Check sheet for the modelled part. Datum: model origin and axes. Units: mm. A direction names the side the tool comes from. Round coordinates to 2 decimals unless told otherwise and drop trailing zeros. Write each loop counter-clockwise with the first axis right and the second up, starting at its lowest first coordinate (ties: lowest second). Pieces come first, ordered by that corner, then holes. Notation, with made-up numbers: (0.5, 3) -> (55.5, 3) arc R6 ccw to (55.5, 9) -> close; hole circle Ø5 at (30.25, 17.5). An arc over 180 degrees is marked (long way). Put each result on its own line as item: value. Start each with the question number.
from build123d import *

# Parameters (mm, degrees)
IZIM1_R                     = 45
Y_KSEKLIK_EKSTR_ZYON1_DEPTH = 35
IZIM2_W                     = 34
IZIM2_H                     = 34
KES_EKSTR_ZYON1_DEPTH       = 4
IZIM5_R                     = 12
KES_EKSTR_ZYON2_DEPTH       = 107.536378763
KES_EKSTR_ZYON3_DEPTH       = 19
IZIM8_R                     = 45
IZIM8_R_2                   = 43
KES_EKSTR_ZYON4_DEPTH       = 1.5
KES_EKSTR_ZYON5_REACH       = 108.536
IZIM9_R                     = 1.5
DAIRESEL_KAPLAMA1_COUNT     = 6


with BuildPart() as part:
    # Çizim1 → Yükseklik-Ekstrüzyon1 (new, symmetric)
    with BuildSketch(Plane(origin=(0, 0, 0), x_dir=(1, 0, 0), z_dir=(0, 1, 0))):
        with Locations(Location((0, 0, 0), (0, 0, 270))):
            Circle(IZIM1_R)
    extrude(amount=Y_KSEKLIK_EKSTR_ZYON1_DEPTH, both=True)

    # Çizim2 → Kes-Ekstrüzyon1 (cut)
    with BuildSketch(Plane.XY.offset(45)):
        with Locations((0, -10)):
            Rectangle(IZIM2_W, IZIM2_H)
    kes_ekstr_zyon1 = extrude(amount=-KES_EKSTR_ZYON1_DEPTH, mode=Mode.SUBTRACT)

    # Aynalama1: Kes-Ekstrüzyon1 across plane
    add(kes_ekstr_zyon1.mirror(Plane.XY), mode=Mode.SUBTRACT)

    # Çizim5 → Kes-Ekstrüzyon2 (cut, through all)
    with BuildSketch(Plane.XY.offset(45)):
        with Locations((0, -10)):
            Circle(IZIM5_R)
    extrude(amount=-KES_EKSTR_ZYON2_DEPTH, mode=Mode.SUBTRACT)

    # Çizim7 → Kes-Ekstrüzyon3 (cut, symmetric)
    with BuildSketch(Plane(origin=(0, 0, 0), x_dir=(0, 0, -1), z_dir=(1, 0, 0))):
        with BuildLine():
            Line((38, -35), (38, -27))
            Line((38, -27), (12, -27))
            Line((12, -27), (12, 11))
            Line((12, 11), (38, 11))
            Line((38, 11), (38, 26))
            ThreePointArc((38, 26), (37.414213562, 27.414213562), (36, 28))
            Line((36, 28), (-36, 28))
            ThreePointArc((-36, 28), (-37.414213562, 27.414213562), (-38, 26))
            Line((-38, 26), (-38, 11))
            Line((-38, 11), (-11.999999881, 11))
            Line((-11.999999881, 11), (-11.999999881, -27))
            Line((-11.999999881, -27), (-38, -27))
            Line((-38, -27), (-38, -35))
            Line((-38, -35), (38, -35))
        make_face()
    extrude(amount=KES_EKSTR_ZYON3_DEPTH, both=True, mode=Mode.SUBTRACT)

    # Çizim8 → Kes-Ekstrüzyon4 (cut, symmetric)
    with BuildSketch(Plane(origin=(0, 23.5, 0), x_dir=(1, 0, 0), z_dir=(0, 1, 0))):
        with Locations(Location((0, 0, 0), (0, 0, 270))):
            Circle(IZIM8_R)
        with Locations(Location((0, 0, 0), (0, 0, 270))):
            Circle(IZIM8_R_2, mode=Mode.SUBTRACT)
    extrude(amount=KES_EKSTR_ZYON4_DEPTH, both=True, mode=Mode.SUBTRACT)

    # Çizim9 → Kes-Ekstrüzyon5 (cut, up to next)
    with BuildSketch(Plane.XY.offset(45), mode=Mode.PRIVATE) as kes_ekstr_zyon5_sk1:
        with Locations(Location((0, 23.5, 0), (0, 0, 90))):
            Circle(IZIM9_R)
    kes_ekstr_zyon5_tool1 = extrude(kes_ekstr_zyon5_sk1.sketch, amount=-KES_EKSTR_ZYON5_REACH, mode=Mode.PRIVATE) & part.part
    kes_ekstr_zyon5 = kes_ekstr_zyon5_tool1.solids().sort_by_distance((0, 23.5, 45))[0]
    add(kes_ekstr_zyon5, mode=Mode.SUBTRACT)

    # Dairesel Kaplama1: Kes-Ekstrüzyon5; each copy of Kes-Ekstrüzyon5 runs up to whatever stops it at its own place
    dairesel_kaplama1_before = part.part  # the part as the pattern finds it: every copy runs up to it
    dairesel_kaplama1_kes_ekstr_zyon5_long = extrude(kes_ekstr_zyon5_sk1.sketch, amount=-KES_EKSTR_ZYON5_REACH, mode=Mode.PRIVATE)
    dairesel_kaplama1_kes_ekstr_zyon5_tool = dairesel_kaplama1_kes_ekstr_zyon5_long.rotate(Axis((0, 25, 0), (0, 1, 0)), 1 * 360 / DAIRESEL_KAPLAMA1_COUNT) & dairesel_kaplama1_before
    add(dairesel_kaplama1_kes_ekstr_zyon5_tool.solids().sort_by_distance((38.971143, 23.5, 22.5))[0], mode=Mode.SUBTRACT)
    dairesel_kaplama1_kes_ekstr_zyon5_tool = dairesel_kaplama1_kes_ekstr_zyon5_long.rotate(Axis((0, 25, 0), (0, 1, 0)), 2 * 360 / DAIRESEL_KAPLAMA1_COUNT) & dairesel_kaplama1_before
    add(dairesel_kaplama1_kes_ekstr_zyon5_tool.solids().sort_by_distance((38.971143, 23.5, -22.5))[0], mode=Mode.SUBTRACT)
    dairesel_kaplama1_kes_ekstr_zyon5_tool = dairesel_kaplama1_kes_ekstr_zyon5_long.rotate(Axis((0, 25, 0), (0, 1, 0)), 3 * 360 / DAIRESEL_KAPLAMA1_COUNT) & dairesel_kaplama1_before
    add(dairesel_kaplama1_kes_ekstr_zyon5_tool.solids().sort_by_distance((0, 23.5, -45))[0], mode=Mode.SUBTRACT)
    dairesel_kaplama1_kes_ekstr_zyon5_tool = dairesel_kaplama1_kes_ekstr_zyon5_long.rotate(Axis((0, 25, 0), (0, 1, 0)), 4 * 360 / DAIRESEL_KAPLAMA1_COUNT) & dairesel_kaplama1_before
    add(dairesel_kaplama1_kes_ekstr_zyon5_tool.solids().sort_by_distance((-38.971143, 23.5, -22.5))[0], mode=Mode.SUBTRACT)
    dairesel_kaplama1_kes_ekstr_zyon5_tool = dairesel_kaplama1_kes_ekstr_zyon5_long.rotate(Axis((0, 25, 0), (0, 1, 0)), 5 * 360 / DAIRESEL_KAPLAMA1_COUNT) & dairesel_kaplama1_before
    add(dairesel_kaplama1_kes_ekstr_zyon5_tool.solids().sort_by_distance((-38.971143, 23.5, 22.5))[0], mode=Mode.SUBTRACT)


solid = part.part
1. Section check B-B, the plane z = 0. Enter the section's corners in (x, y), then the cut area to 3 significant figures.
2. Section check C-C, the plane y = -24. Enter the section's corners in (x, z).
3. Access from +Z, -Z, +X, -X, +Y, -Y to the whole of each face (thin tool, end or side, straight path). Record for faces 4 (the flat face through (-36.5, 25, 23.1)), 5 (the flat face through (-8, 1, 12)), 6 (the flat face through (0, -27, 43)), 7 (the flat face through (0, 7, -43)).
4. Section check D-D, the plane y = 23.5. Enter the section's corners in (x, z).
5. Draft check along X on faces 1 (the cylindrical face through (-43.93, -6.1, -9.76)), 2 (the flat face through (0, 18, -38)), 3 (the cylindrical face through (-21.77, 23.48, 37.08)). Enter one of: released by +X, released by -X, zero draft, split by the parting line, or undercut.
6. Section check A-A, the plane y = -10. Enter the section's corners in (x, z), then the cut area to 3 significant figures.
7. Material ranges on L1, parallel to Y at x = 0, z = 23; L2, parallel to X at y = -2, z = -32; L3, parallel to X at y = -18, z = -33.5, recorded low to high. Write a range as [from, to].
8. Gauge pin test, flat ends, axial feed: P1, Ø1.5, axis at x = 9, y = -0.5, coming from the +Z side; P2, Ø19, axis at y = 1.5, z = 17.5, coming from the -X side; P3, Ø1, axis at x = 17, y = -0.5, coming from the -Z side; P4, Ø2.5, axis at x = 0, y = 23.5, coming from the +Z side. Record the tip position at first contact, or that the pin passes through.
Reply:
1. outline: (-45, -35) -> (-19, -35) -> (-19, 28) -> (19, 28) -> (19, -35) -> (45, -35) -> (45, 22) -> (43, 22) -> (43, 25) -> (45, 25) -> (45, 35) -> (-45, 35) -> (-45, 25) -> (-43, 25) -> (-43, 22) -> (-45, 22) -> close
1. area: 3,890 mm2
2. outline: (-17, -41.67) -> (-17, -41) -> (17, -41) -> (17, -41.67) arc R45 ccw to (17, 41.67) -> (17, 41) -> (-17, 41) -> (-17, 41.67) arc R45 ccw to start; hole (-19, -12) -> (19, -12) -> (19, 12) -> (-19, 12) -> close
3. face 4: none
3. face 5: -Y
3. face 6: +Z
3. face 7: -Z
4. outline: (-37.97, -20.19) -> (-19, -9.24) -> (-19, 9.24) -> (-37.97, 20.19) arc R43 ccw to start; (-36.47, -22.79) arc R43 ccw to (-1.5, -42.97) -> (-1.5, -38) -> (-19, -38) -> (-19, -12.7) -> close; (-36.47, 22.79) -> (-19, 12.7) -> (-19, 38) -> (-1.5, 38) -> (-1.5, 42.97) arc R43 ccw to start; (1.5, -42.97) arc R43 ccw to (36.47, -22.79) -> (19, -12.7) -> (19, -38) -> (1.5, -38) -> close; (1.5, 38) -> (19, 38) -> (19, 12.7) -> (36.47, 22.79) arc R43 ccw to (1.5, 42.97) -> close; (19, -9.24) -> (37.97, -20.19) arc R43 ccw to (37.97, 20.19) -> (19, 9.24) -> close
5. face 1: split by the parting line
5. face 2: undercut
5. face 3: released by -X
6. outline: (-19, -12) -> (-19, 12) -> (-12, 12) -> (-12, 41) -> (-17, 41) -> (-17, 41.67) arc R45 ccw to (-17, -41.67) -> (-17, -41) -> (-12, -41) -> (-12, -12) -> close; (12, -41) -> (17, -41) -> (17, -41.67) arc R45 ccw to (17, 41.67) -> (17, 41) -> (12, 41) -> (12, 12) -> (19, 12) -> (19, -12) -> (12, -12) -> close
6. area: 3,860 mm2
7. L1: y = [-27, -22], [2, 11], [28, 35]
7. L2: x = [-31.64, -8.94], [8.94, 31.64]
7. L3: x = [-30.05, -8.94], [8.94, 30.05]
8. P1: stops at z = 41
8. P2: stops at x = -44.28
8. P3: stops at z = -41.67
8. P4: passes through
